Job drawing, mm, ordinate dimensions from the low corner. One solid piece. A direction names the side the tool comes from. Coordinates: 2 decimals unless noted, no trailing zeros. Order: outer loops, then holes, each group sorted by start corner. A loop starts at its lowest first (then second) coordinate and runs counter-clockwise, first axis right, second up. Notation, with made-up numbers: (13.5, 24) - (59.5, 24) arc R18 cw to (59.5, 59) - close; hole circle Ø1 at (87, 85). An arc over 180 degrees is marked (long way). Use a Markdown table: item, result. Add a question column.
1) Saw through at C-C on x = 7.5. List the corners of the cut face in (y, z).
2) Saw through at B-B on y = 74. List the corners of the cut face in (x, z).
3) Drop flat-ended pins along their axis: P1, Ø2, axis at x = 42.5, z = 10.5, coming from the +Y side; P2, Ø5, axis at y = 43.5, z = 8.5, coming from the +X side (3 decimals); P3, Ø6.5, axis at x = 40, y = 40, coming from the +Z side; P4, Ø8, axis at x = 31.5, z = 19, coming from the +Y side. Give the stop position or say it passes through.
4) Tool access for the marked faces 1 and 2: list every direction of +Z, -Z, +X, -X, +Y, -Y with a clear straight run to the whole face (end or side of a thin tool).
5) Wall check: L1, parallel to Y at x = 40, z = 20.4; L2, parallel to Z at x = 69, y = 29; L3, parallel to Z at x = 46, y = 40. Give the ranges that are in metal, low to high. Write a range as [from, to].
6) Two-plate mould, pull along X, no slides. Class the marked faces 3, 4 and 5: +X half, -X half, draft (parallel to the pull), parting line (faces both ways), or undercut.
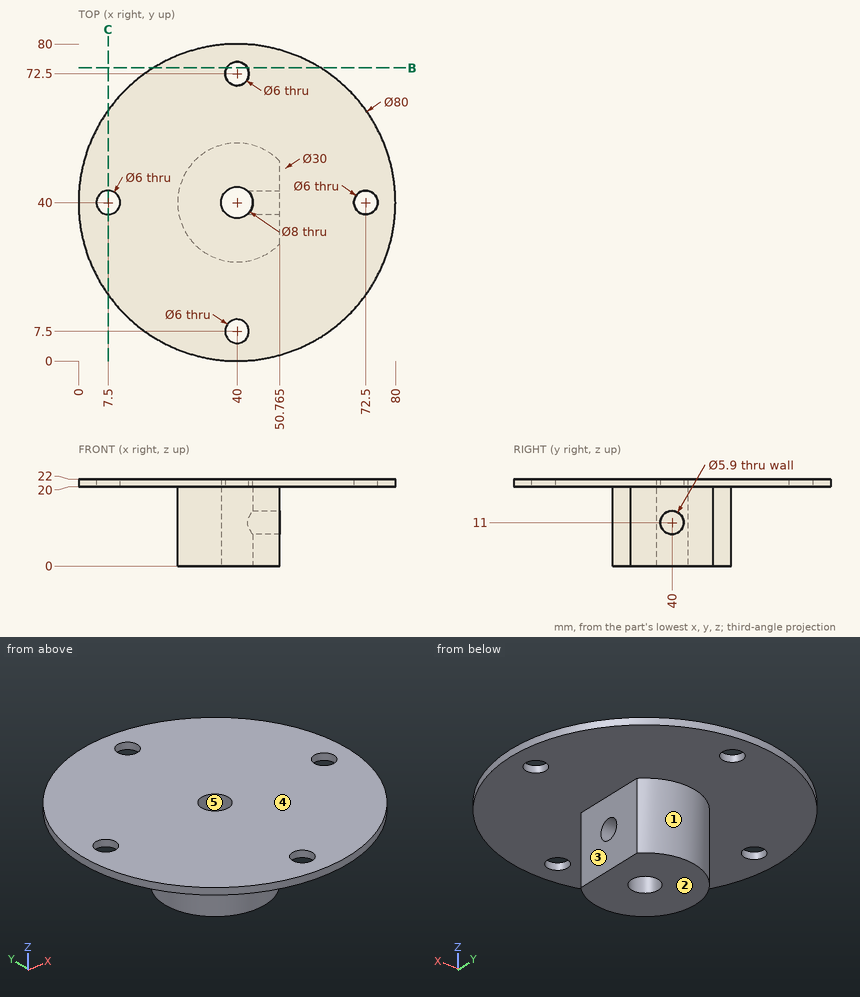
Results are:
| question | item | result |
|---|---|---|
| 1 | outline | (16.68, 20) - (37, 20) - (37, 22) - (16.68, 22) - close; (43, 20) - (63.32, 20) - (63.32, 22) - (43, 22) - close |
| 2 | outline | (18.93, 20) - (37.4, 20) - (37.4, 22) - (18.93, 22) - close; (42.6, 20) - (61.07, 20) - (61.07, 22) - (42.6, 22) - close |
| 3 | P1 | y = 54.92 |
| 3 | P2 | x = 50.765 |
| 3 | P3 | through |
| 3 | P4 | y = 79.73 |
| 4 | face 1 | -Z |
| 4 | face 2 | -Z, +X, -X, +Y, -Y |
| 5 | L1 | [0, 4.5], [10.5, 36], [44, 69.5], [75.5, 80] |
| 5 | L2 | [20, 22] |
| 5 | L3 | [0, 8.05], [13.95, 22] |
| 6 | face 3 | +X half |
| 6 | face 4 | draft |
| 6 | face 5 | undercut |
